Source: CAD feature listing. Evaluate the final solid. Frame: model axes, mm. Give positions to 0.01 mm unless a question says otherwise; leave off trailing zeros. Loops run counter-clockwise (first coordinate to the right, second up) from the corner with the lowest first, then second, coordinate; pieces in that order, holes last. Notation, with made-up numbers: (-11, 35) -> (27, 35) arc R12 ccw to (27, 50) -> close; hole circle Ø9 at (25.25, -38.75). An arc over 180 degrees is marked (long way). Return JSON: item names as keys, results as strings. Group by question number.
(1) Cut plane D-D on x = -8. Return loops of the section in (y, z).
(2) Pin query (flat end, axial travel): pin 1 (1.2 mm diameter, centred on x = -9.5, z = -2, fed in from -Y). Return the tip coordinate at first contact, or that it passes through.
(3) Draft query along Z for faces 1 (the face through (-8.94, 3.4, -7.76)), 2 (the face through (-9, 2, -2)), 3 (the face through (-10.5, 0.99, -0.98)), 4 (the face through (-3.023, 1, -2)). Return one class per face: released by +Z, released by -Z, zero draft, split by the parting line, or undercut.
(4) Cut plane B-B on z = 0.5. Return loops of the section in (x, y).
(5) Ray query, line 1 (X direction, y = 2.1, z = -5.75); line 2 (X direction, y = 0.4, z = -2); line 3 (X direction, y = 0.6, z = -3.5). Return the intervals inside material, ascending. Write a range as from..to.
(6) Cut plane C-C on y = 0.45. Return loops of the section in (x, z).
(7) Cut plane A-A on x = -12.5. Return loops of the section in (y, z), then the cut area to 3 significant figures.
```python
from build123d import *

# Parameters (mm, degrees)
SKETCH1_W           = 12
SKETCH1_H           = 12
BOSS_EXTRUDE1_DEPTH = 4
SKETCH2_R           = 2
CUT_EXTRUDE1_DEPTH  = 2
FILLET1_R           = 2


with BuildPart() as part:
    # Sketch1 → Boss-Extrude1 (new body)
    with BuildSketch(Plane(origin=(0, 0, 0), x_dir=(1, 0, 0), z_dir=(0, 1, 0))):
        with Locations((-9.023076923, 2.330769231)):
            Rectangle(SKETCH1_W, SKETCH1_H)
    extrude(amount=BOSS_EXTRUDE1_DEPTH)

    # Sketch2 → Cut-Extrude1 (cut)
    with BuildSketch(Plane.XZ):
        with Locations((-9.023076923, -2.330769231)):
            Circle(SKETCH2_R)
    extrude(amount=-CUT_EXTRUDE1_DEPTH, mode=Mode.SUBTRACT)

    # Fillet1
    fillet1_edges = [part.edges().sort_by_distance(p)[0] for p in [
        (-15.023076923, 4, -2.330769231),
        (-9.023076923, 4, 3.669230769),
        (-3.023076923, 4, -2.330769231),
        (-9.023076923, 4, -8.330769231),
    ]]
    fillet(fillet1_edges, radius=FILLET1_R)


solid = part.part
```
Answers:
{
 "1": {"outline": "(0, -8.33) -> (2, -8.33) arc R2 ccw to (4, -6.33) -> (4, 1.67) arc R2 ccw to (2, 3.67) -> (0, 3.67) -> (0, -0.61) -> (2, -0.61) -> (2, -4.05) -> (0, -4.05) -> close"},
 "2": {"pin 1": "y = 2"},
 "3": {"face 1": "released by -Z", "face 2": "undercut", "face 3": "undercut", "face 4": "zero draft"},
 "4": {"outline": "(-15.02, 0) -> (-3.02, 0) -> (-3.02, 2) arc R2 ccw to (-5.02, 4) -> (-13.02, 4) arc R2 ccw to (-15.02, 2) -> close"},
 "5": {"line 1": "-15.02..-3.03", "line 2": "-15.02..-11, -7.05..-3.02", "line 3": "-15.02..-10.65, -7.4..-3.02"},
 "6": {"outline": "(-15.02, -8.33) -> (-3.02, -8.33) -> (-3.02, 3.67) -> (-15.02, 3.67) -> close; hole circle Ø4 at (-9.02, -2.33)"},
 "7": {"outline": "(0, -8.33) -> (2, -8.33) arc R2 ccw to (4, -6.33) -> (4, 1.67) arc R2 ccw to (2, 3.67) -> (0, 3.67) -> close", "area": "46.3 mm²"}
}
